Geometry: final body of the model. Coordinates: model frame, mm. A direction names the side the tool comes from. Round coordinates to 2 decimals unless told otherwise and drop trailing zeros. Order: outer loops, then holes, each group sorted by start corner. A loop starts at its lowest first (then second) coordinate and runs counter-clockwise, first axis right, second up. Notation, with made-up numbers: M 10.5,-37 L 19.5,-37 A13 ccw 19.5,-28 Z; hole C 31,-21.75 d7. An arc over 180 degrees is marked long. Put each result on its own line as item: value. Start each with the question number.
1) Material intervals for probe 1 along Z at (x, y) = (9, 33); probe 2 along Z at (x, y) = (24.5, 33); probe 3 along X at (y, z) = (18, 14), sorted ascending. Write a range as [from, to].
2) Draft query along Z for faces 3 (the flat face through (15, 45, 31.5)), 4 (the flat face through (12, 42, 14)), 5 (the flat face through (0, 52, 14)). Return one class per face: pulls with the +Z half, pulls with the -Z half, needs draft (parallel to the pull), parting line crosses it, or undercut.
3) Section C-C, the plane y = 33. Return loops of the section in (x, z), then the cut area to 3 significant figures.
4) First-contact query: P1, Ø21, axis at y = 23, z = -0.5, coming from the -X side; P2, Ø3, axis at x = 12, z = 5.5, coming from the +Y side; P3, Ø1.5, axis at x = 18.5, z = -21, coming from the -Y side; P4, Ø8, axis at x = 15, y = 72.6, coming from the +Z side. Flat tips, straight axial feed; report the tip coordinate or a pass-through.
5) Section D-D, the plane x = 27.5. Return loops of the section in (y, z).
6) Section B-B, the plane z = 0. Return loops of the section in (x, y).
7) Section A-A, the plane x = 15. Return loops of the section in (y, z).
8) Access query for faces 1 (the cylindrical face through (21.126, 18.128, -1.953)), 2 (the cylindrical face through (6.08, 51.63, 9.69)). Directions: +Z, -Z, +X, -X, +Y, -Y. A direction counts if a zero-diameter tool reaches every point of the face in a straight line with its end or side. Return the directions, or none.
Autodesk Inventor part; units mm, degrees
ref_plane "YZ Plane" through (0, 0, 0) normal (1, 0, 0) x (0, 1, 0)
ref_plane "XZ Plane" through (0, 0, 0) normal (0, 1, 0) x (-1, 0, 0)
ref_plane "XY Plane" through (0, 0, 0) normal (0, 0, 1) x (1, 0, 0)
sketch "Sketch1" plane through (0, 0, 0) normal (1, 0, 0) x (0, 1, 0)
  arc A0 (4.6958, 31.5) -> (4.6958, -31.5) centre (108, 0) ccw
  line L0 (4.6958, 31.5) -> (85.6007, 31.5)
  line L1 (85.6007, 31.5) -> (85.6007, -31.5)
  line L2 (85.6007, -31.5) -> (4.6958, -31.5)
  point P0 (0, 0)
  point P1 (0, 0)
  point P2 (4.6958, -31.5)
  dimension "d0" = 108
  dimension "d1" = 63
  dimension "d2" = 0
extrude "Extrusion1" add sketch "Sketch1" along normal blind 30
fillet "Fillet1" radius 13 1 edges at (0, 85.6007, 0)
sketch "Sketch2" plane through (0, 4.6958, 31.5) normal (0, 0, 1) x (1, 0, 0)
  circle A0 centre (15, 67.9049) radius 6.5
  line L0 (13, 80.9049) -> (30, 80.9049)
  line L1 (30, 80.9049) -> (30, 0)
  point P0 (0, -4.6958)
  dimension "d7" = 13
  dimension "d8" = 15
  dimension "d9" = 13
extrude "Extrusion2" cut sketch "Sketch2" against normal through all
sketch "Sketch3" plane through (0, 0, 0) normal (-1, 0, 0) x (0, 0, 1)
  point P0 (0, 0)
  point P1 (0, 33)
  dimension "d12" = 33
hole "Hole1" at (0, 33, 0) direction (1, 0, 0) diameter 30 end through all counterbore diameter 42 counterbore depth 12
properties part number "drag release plate"
Result sheet:
1. probe 1: z = [-31.5, -21], [21, 31.5]
1. probe 2: z = [-31.5, -15], [15, 31.5]
1. probe 3: x = [12, 30]
2. face 3: pulls with the +Z half
2. face 4: undercut
2. face 5: needs draft
3. outline: M 0,-31.5 L 30,-31.5 L 30,-15 L 12,-15 L 12,-21 L 0,-21 Z; M 0,21 L 12,21 L 12,15 L 30,15 L 30,31.5 L 0,31.5 Z
3. area: 846 mm2
4. P1: stops at x = 12
4. P2: stops at y = 85.6
4. P3: stops at y = 1.92
4. P4: passes through
5. outline: M 4.7,-31.5 L 85.6,-31.5 L 85.6,31.5 L 4.7,31.5 A108 ccw Z; hole C 33,0 d30
6. outline: M 0,0 L 30,0 L 30,18 L 12,18 L 12,12 L 0,12 Z; M 0,54 L 12,54 L 12,48 L 30,48 L 30,85.6 L 13,85.6 A13 ccw 0,72.6 Z; hole C 15,72.6 d13
7. outline: M 4.7,-31.5 L 66.1,-31.5 L 66.1,31.5 L 4.7,31.5 A108 ccw Z; M 79.1,-31.5 L 85.6,-31.5 L 85.6,31.5 L 79.1,31.5 Z; hole C 33,0 d30
8. face 1: +X, -X
8. face 2: -X
